from build123d import *

# Parameters (mm, degrees)
F0_R     = 139.7
F1_DEPTH = 12.7
F6_D     = 6.35
F6_DEPTH = 50.8
F6_TIP   = 1.9077324654


# Not quite as in the source:
# - a pattern or mirror of a feature is missing from the dataset's text; its kind, count and spacing are read off the source's solid


with BuildPart() as f1:
    # F0 (on Front) → F1 (new body)
    with BuildSketch(Plane.XZ):
        with BuildLine():
            ThreePointArc((15.8551438321, -157.95625), (0, 158.75), (-15.8551438321, -157.95625))
            Line((-15.8551438321, -157.95625), (15.8551438321, -157.95625))
        make_face()
        Circle(F0_R, mode=Mode.SUBTRACT)
    extrude(amount=F1_DEPTH)

    # F6
    with Locations(Plane(origin=(0, 0, 0), x_dir=(1, 0, 0), z_dir=(0, 1, 0))):
        with Locations((38.6222720054, -144.140281428)):
            f6 = Hole(F6_D / 2, depth=F6_DEPTH)
            with Locations((0, 0, -(F6_DEPTH + F6_TIP / 2))):  # 118° drill point
                Cone(0, F6_D / 2, F6_TIP, mode=Mode.SUBTRACT)

    # F6_copies: F6 across plane
    add(f6.mirror(Plane(origin=(0, 0, 0), x_dir=(-0.9659258263, 0, 0.2588190451), z_dir=(-0.2588190451, 0, -0.9659258263))), mode=Mode.SUBTRACT)


solid = f1.part
The model under review builds one solid part; all positions refer to its coordinate system, in mm. Give positions to 0.01 mm unless a question says otherwise; leave off trailing zeros. Order: outer loops, then holes, each group sorted by start corner. A loop starts at its lowest first (then second) coordinate and runs counter-clockwise, first axis right, second up. Notation, with made-up numbers: M 58,22.25 L 98,22.25 A22 cw 98,51.25 Z; hole C 59,19 d2. An arc over 180 degrees is marked long. Answer in a Markdown table with one row per item. Add a question column.
1. Add section A-A on x = 0. State the section outline as (y, z) points, plus the area to 3 significant figures.
2. For pin 1 Ø4 at (x, y) = (-73.5, -6.5) entering from -Z; pin 2 Ø5 at (y, z) = (-3.5, 43.5) entering from -X; pin 3 Ø5 at (y, z) = (-8.5, 71) entering from -X, all flat-tipped, find the tip position at first contact; note any pin that passes through.
3. Add section B-B on z = 0. State the section outline as (x, y) points, plus the area to 3 significant figures.
4. To check wall thickness, follow line 1 along X through (y, z) = (-6, -3.5); line 2 along X through (y, z) = (-3.5, 56); line 3 along Z through (x, y) = (63.5, -10.75). State the ranges of each line that lie inside material, in increasing order.
5. Add section C-C on y = -8.5. State the section outline as (x, z) points (3 decimals).
6. Mouldability with a two-part tool opening along X and no side actions: class faces 1 (the cylindrical face through (6.758, -6.261, 158.606)), 2 (the cylindrical face through (-110.86, -6.26, -85.01)), 3 (the flat face through (105, -12.7, -93)) as released by +X, released by -X, zero draft, split by the parting line, or undercut.
The answers:
| question | item | result |
|---|---|---|
| 1 | outline | M -12.7,-157.96 L 0,-157.96 L 0,-139.7 L -12.7,-139.7 Z; M -12.7,139.7 L 0,139.7 L 0,158.75 L -12.7,158.75 Z |
| 1 | area | 474 mm2 |
| 2 | pin 1 | z = -141.74 |
| 2 | pin 2 | x = -153.36 |
| 2 | pin 3 | x = -143.21 |
| 3 | outline | M -158.75,-12.7 L -139.7,-12.7 L -139.7,0 L -158.75,0 Z; M 139.7,-12.7 L 158.75,-12.7 L 158.75,0 L 139.7,0 Z |
| 3 | area | 484 mm2 |
| 4 | line 1 | -158.71 to -139.66, 139.66 to 158.71 |
| 4 | line 2 | -148.54 to -127.98, 127.98 to 148.54 |
| 4 | line 3 | -145.5 to -124.43, 124.43 to 145.5 |
| 5 | outline | M -15.855,-157.956 L 15.855,-157.956 A158.75 ccw long Z; hole C 0,0 d279.4; hole C -38.622,-144.14 d6.35; hole C 38.622,144.14 d6.35 |
| 6 | face 1 | split by the parting line |
| 6 | face 2 | undercut |
| 6 | face 3 | zero draft |
